Autodesk Inventor part; units mm, degrees
ref_plane "YZ Plane" through (0, 0, 0) normal (1, 0, 0) x (0, 1, 0)
ref_plane "XZ Plane" through (0, 0, 0) normal (0, 1, 0) x (-1, 0, 0)
ref_plane "XY Plane" through (0, 0, 0) normal (0, 0, 1) x (1, 0, 0)
sketch "Sketch1" plane through (0, 0, 0) normal (0, 1, 0) x (-1, 0, 0)
  arc A0 (0, 9.75) -> (0, -9.75) centre (0, 0) ccw
  arc A1 (0, 6) -> (0, -6) centre (0, 0) ccw
  line L0 (0, 9.75) -> (0, 12.75)
  line L1 (0, -9.75) -> (0, -12.75)
  line L2 (0, -12.75) -> (-12, -12.75)
  line L3 (-12, -12.75) -> (-12, 12.75)
  line L4 (-12, 12.75) -> (0, 12.75)
  line L5 (0, 9.75) -> (0, -9.75)
  dimension "d0" = 19.5
  dimension "d1" = 12
  dimension "d2" = 3
  dimension "d3" = 3
  dimension "d4" = 12
extrude "Extrusion4" add sketch "Sketch1" along normal blind 11 and the other way blind 6.5 contours L5 A1 A0 | A0 L1 L2 L3 L4 L0
extrude "Extrusion5" cut sketch "Sketch1" along normal blind 3 and the other way blind 3.5 contours L5 A1 A0
sketch "Sketch3" plane through (0, -6.5, 12.75) normal (-1, 0, 0) x (0, 0, 1)
  line L0 (-25.5, 17.5) -> (-18.75, 17.5)
  line L1 (-22.125, 17.5) -> (-22.125, 9.5)
  line L2 (-3, 9.5) -> (-22.5, 9.5)
  line L3 (0, 17.5) -> (-6.75, 17.5)
  line L4 (-6.75, 17.5) -> (0, 17.5)
  line L5 (-3.375, 17.5) -> (-3.375, 9.5)
  circle A0 centre (-22.125, 13.5) radius 2.6
  circle A1 centre (-3.375, 13.5) radius 2.6
  point P0 (-12.75, 6.5)
  dimension "d23" = 5.2
  dimension "d24" = 5.2
extrude "Extrusion6" cut sketch "Sketch3" against normal blind 30
properties part number "bearing_holder"
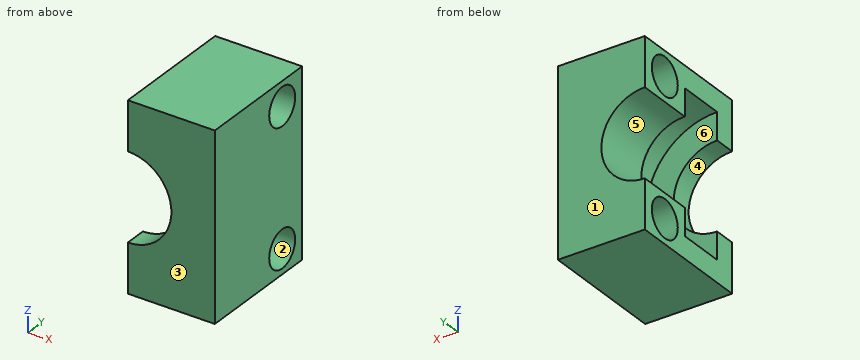
Design review of the part built by this model. Coordinates are the model's own, in mm. Face numbers are marked on the shaded views. A direction names the side the tool comes from. Give positions to 0.01 mm unless a question says otherwise; leave off trailing zeros. Order: outer loops, then holes, each group sorted by start corner. A loop starts at its lowest first (then second) coordinate and runs counter-clockwise, first axis right, second up.
1. Add section C-C, the plane x = 5. State the section outline as (y, z) points (3 decimals).
Solution:
outline: (-6.5, -12.75) - (11, -12.75) - (11, -3.317) - (3, -3.317) - (3, -8.37) - (-3.5, -8.37) - (-3.5, -3.317) - (-6.5, -3.317) - close; (-6.5, 3.317) - (-3.5, 3.317) - (-3.5, 8.37) - (3, 8.37) - (3, 3.317) - (11, 3.317) - (11, 12.75) - (-6.5, 12.75) - close; hole circle Ø5.2 at (7, -9.375); hole circle Ø5.2 at (7, 9.375)
2. To check wall thickness, follow L1, parallel to Z at x = 9, y = 7 (3 decimals); L2, parallel to Y at x = 7.5, z = 4; L3, parallel to Y at x = 0.5, z = 8.5. State the ranges of each line that lie inside material, in increasing order.
Solution:
L1: z = -12.75 to -11.975, -6.775 to 6.775, 11.975 to 12.75
L2: y = -6.5 to -3.5, 3 to 11
L3: y = -6.5 to -3.5, 3 to 4.55, 9.45 to 11
3. Add section A-A, the plane y = 7. State the section outline as (x, z) points (3 decimals).
Solution:
outline: (0, -12.75) - (12, -12.75) - (12, -11.975) - (0, -11.975) - close; (0, -6.775) - (12, -6.775) - (12, 6.775) - (0, 6.775) - (0, 6) arc R6 cw to (0, -6) - close; (0, 11.975) - (12, 11.975) - (12, 12.75) - (0, 12.75) - close
4. For pin 1 Ø2 at (y, z) = (8.5, 1) entering from -X, flat-tipped, find the tip position at first contact; note if it passes through.
Solution:
pin 1: stops at x = 5.66
5. Tool access review of the marked faces 5 and 6: name each direction out of +Z, -Z, +X, -X, +Y, -Y from which nothing blocks a thin tool from reaching the whole face with its end or side.
Solution:
face 5: -X, +Y, -Y
face 6: -X
6. Mouldability with a two-part tool opening along Y and no side actions: class the marked faces 1, 2, 3 and 4 as +Y half, -Y half, draft (parallel to the pull), parting line (faces both ways), or undercut.
Solution:
face 1: +Y half
face 2: undercut
face 3: -Y half
face 4: draft
7. Add section B-B, the plane z = 0. State the section outline as (x, y) points, then the cut area to 3 significant figures.
Solution:
outline: (6, -6.5) - (12, -6.5) - (12, 11) - (6, 11) - (6, 3) - (9.75, 3) - (9.75, -3.5) - (6, -3.5) - close
area: 80.6 mm2
8. Add section D-D, the plane y = 2.25. State the section outline as (x, z) points, then the cut area to 3 significant figures.
Solution:
outline: (0, -12.75) - (12, -12.75) - (12, 12.75) - (0, 12.75) - (0, 9.75) arc R9.75 cw to (0, -9.75) - close
area: 157 mm2
